Design review of the part shown in the three views and the two pictorial views. Dimensions are in mm from the part's minimum x, y and z. Round coordinates to 2 decimals unless told otherwise and drop trailing zeros. Order: outer loops, then holes, each group sorted by start corner. A loop starts at its lowest first (then second) coordinate and runs counter-clockwise, first axis right, second up. Notation, with made-up numbers: M 89.25,36 L 128.25,36 A27 cw 128.25,58 Z; hole C -35,30 d1. An arc over 180 degrees is marked long. Use a Markdown table: item, result. Add a question column.
(1) The part is to be moulded in two halves that separate along X. For the marked faces 1, 2, 3 and 4, say which applies: released by +X, released by -X, zero draft, split by the parting line, or undercut.
(2) Take a section at A-A (z = 1.6). Write out the cut boundary in (x, y), then the cut area to 3 significant figures.
(3) For pin 1 (4.5 mm diameter, centred on x = 4, y = 4.62, fed in from -Z); pin 2 (1 mm diameter, centred on x = 7, y = 8, fed in from +Z), all flat-tipped, find the tip position at first contact; note any pin that passes through.
(4) To check wall thickness, follow probe 1 along X at (y, z) = (4.5, 0.8); probe 2 along X at (y, z) = (6, 1.45) (1 decimal); probe 3 along Y at (x, z) = (3.25, 2.05) (1 decimal). State the ranges of each line that lie inside material, in increasing order. Write a range as from..to.
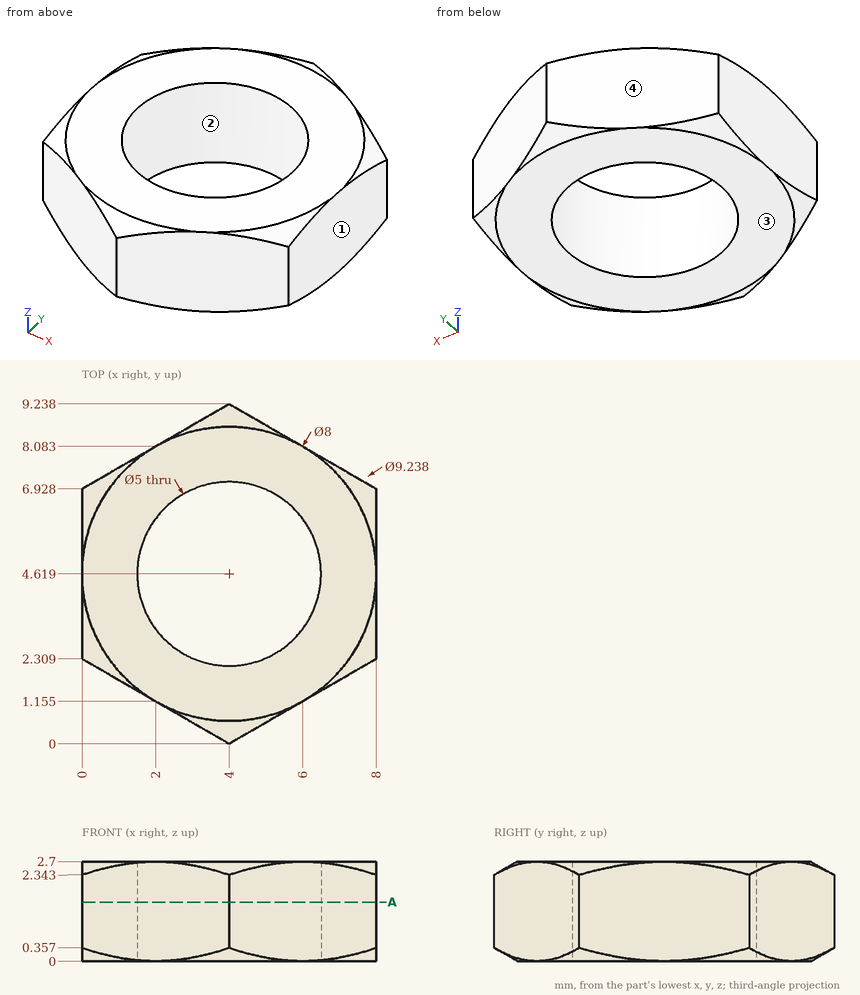
Verdict:
| question | item | result |
|---|---|---|
| 1 | face 1 | released by +X |
| 1 | face 2 | undercut |
| 1 | face 3 | zero draft |
| 1 | face 4 | released by -X |
| 2 | outline | M 0,2.31 L 4,0 L 8,2.31 L 8,6.93 L 4,9.24 L 0,6.93 Z; hole C 4,4.62 d5 |
| 2 | area | 35.8 mm^2 |
| 3 | pin 1 | passes through |
| 3 | pin 2 | stops at z = 2.69 |
| 4 | probe 1 | x = 0..1.5, 6.5..8 |
| 4 | probe 2 | x = 0..1.9, 6.1..8 |
| 4 | probe 3 | y = 0.4..2.2, 7..8.8 |
